CAD build for the part. Positions are in the model's coordinates, mm. A direction names the side the tool comes from. Coordinates: 2 decimals unless noted, no trailing zeros. Loops run counter-clockwise (first coordinate to the right, second up) from the corner with the lowest first, then second, coordinate; pieces in that order, holes last.
1) Saw through at A-A, the plane y = -285.75. Write the cut outline in (x, z).
2) Saw through at C-C, the plane z = -21.5. Write the cut outline in (x, y).
3) Two-plate mould, pull along X, no slides. Class faces 6 (the flat face through (-1, 304.8, 1)), 7 (the cylindrical face through (-66.86, -119.14, 12.52)), 8 (the flat face through (-95.25, -176, 16)): +X half, -X half, draft (parallel to the pull), parting line (faces both ways), or undercut.
4) Which spindle directions (+Z, -Z, +X, -X, +Y, -Y) get a long thin tool onto all of the face, cutting with end or side? Do faces 1 (the flat face through (-70, -92.075, 16)), 2 (the cylindrical face through (64.55, -122.16, 12.52)), 3 (the flat face through (95.25, -176, 16)), 4 (the flat face through (-118.269, 4, -25)), 5 (the flat face through (69, -257.175, 16)). Say none if no direction does.
5) Wall check: line 1 along Y through (x, z) = (57, 2); line 2 along X through (y, z) = (120, 1); line 3 along Y through (x, z) = (69.85, 19.75) (3 decimals). Give the ranges that are in metal, low to high.
6) Saw through at B-B, the plane x = -57.15. Write the cut outline in (y, z) (3 decimals), and give its area (3 significant figures).
7) Pin check, flat tips, straight feed: pin 1 Ø5 at (x, y) = (-37.5, -49.5) entering from +Z; pin 2 Ø21 at (x, z) = (59, 18) entering from -Y (3 decimals); pin 3 Ø15 at (y, z) = (-199.5, 15) entering from +X; pin 4 Ø14.5 at (x, y) = (69.85, -123.825) entering from +Z. Stop position of each tip, or through.
8) Saw through at D-D, the plane y = 93. Write the cut outline in (x, z), and give its area (3 significant figures).
```python
from build123d import *

# Parameters (mm, degrees)
F0_R     = 5.55625
F0_R_2   = 7.14375
F1_DEPTH = 6.35
F2_W     = 6.35
F2_H     = 609.6
F3_DEPTH = 50.8
F4_W     = 50.8
F4_H     = 165.1
F5_DEPTH = 19.05
F6_DEPTH = 25.4
F7_R     = 6.35
F8_DEPTH = 25.4


with BuildPart() as f1:
    # F0 (on Top) → F1 (new body)
    with BuildSketch(Plane.XY):
        Polygon((-124.61875, 304.8), (-124.61875, -304.8), (124.61875, -304.8), (124.61875, 304.8), (0, 304.8), align=None)
        with Locations((-69.85, -225.425)):
            Circle(F0_R, mode=Mode.SUBTRACT)
        with Locations((-69.85, -123.825)):
            Circle(F0_R, mode=Mode.SUBTRACT)
        with BuildLine():
            ThreePointArc((75.40625, -225.425), (69.85, -230.98125), (64.29375, -225.425))
            ThreePointArc((64.29375, -225.425), (69.85, -219.86875), (75.40625, -225.425))
        make_face(mode=Mode.SUBTRACT)
        with BuildLine():
            ThreePointArc((75.40625, -123.825), (69.85, -129.38125), (64.29375, -123.825))
            ThreePointArc((64.29375, -123.825), (69.85, -118.26875), (75.40625, -123.825))
        make_face(mode=Mode.SUBTRACT)
        with Locations((-57.15, 120.65)):
            Circle(F0_R_2, mode=Mode.SUBTRACT)
        with Locations((-57.15, 196.85)):
            Circle(F0_R_2, mode=Mode.SUBTRACT)
        with BuildLine():
            ThreePointArc((64.29375, 120.65), (57.15, 113.50625), (50.00625, 120.65))
            ThreePointArc((50.00625, 120.65), (57.15, 127.79375), (64.29375, 120.65))
        make_face(mode=Mode.SUBTRACT)
        with BuildLine():
            ThreePointArc((64.29375, 196.85), (57.15, 189.70625), (50.00625, 196.85))
            ThreePointArc((50.00625, 196.85), (57.15, 203.99375), (64.29375, 196.85))
        make_face(mode=Mode.SUBTRACT)
    extrude(amount=F1_DEPTH)

    # F2 (on face) → F3 (join)
    with BuildSketch(Plane(origin=(0, 0, 0), x_dir=(1, 0, 0), z_dir=(0, 0, -1))):
        with Locations((-121.44375, 0)):
            Rectangle(F2_W, F2_H)
        with Locations((121.44375, 0)):
            Rectangle(F2_W, F2_H)
    extrude(amount=F3_DEPTH)

    # F4 (on face) → F5 (join)
    with BuildSketch(Plane.XY.offset(6.35)):
        with Locations((-69.85, -174.625)):
            Rectangle(F4_W, F4_H)
        with Locations((69.85, -174.625)):
            Rectangle(F4_W, F4_H)
    extrude(amount=F5_DEPTH)

    # F6 (cut): faces of the model
    f6_faces = [f1.faces().sort_by_distance(p)[0] for p in [
        (-69.85, -123.825, 6.35),
        (-69.85, -225.425, 6.35),
        (69.85, -225.425, 6.35),
        (69.85, -123.825, 6.35),
    ]]
    extrude(f6_faces, amount=-F6_DEPTH, mode=Mode.SUBTRACT)

    # F7 (on face) → F8 (cut)
    with BuildSketch(Plane(origin=(0, 0, 0), x_dir=(1, 0, 0), z_dir=(0, 0, -1))):
        with Locations((-92.86875, 285.75)):
            Circle(F7_R)
        with Locations((92.86875, 285.75)):
            Circle(F7_R)
        with Locations((92.86875, -285.75)):
            Circle(F7_R)
        with Locations((-92.86875, -285.75)):
            Circle(F7_R)
    extrude(amount=-F8_DEPTH, mode=Mode.SUBTRACT)


solid = f1.part
```
Data:
1. outline: (-124.62, -50.8) - (-118.27, -50.8) - (-118.27, 0) - (-99.22, 0) - (-99.22, 6.35) - (-124.62, 6.35) - close; (-86.52, 0) - (86.52, 0) - (86.52, 6.35) - (-86.52, 6.35) - close; (99.22, 0) - (118.27, 0) - (118.27, -50.8) - (124.62, -50.8) - (124.62, 6.35) - (99.22, 6.35) - close
2. outline: (-124.62, -304.8) - (-118.27, -304.8) - (-118.27, 304.8) - (-124.62, 304.8) - close; (118.27, -304.8) - (124.62, -304.8) - (124.62, 304.8) - (118.27, 304.8) - close
3. face 6: draft
3. face 7: undercut
3. face 8: -X half
4. face 1: +Z, +X, -X, +Y
4. face 2: +Z, -Z
4. face 3: +Z, +X, +Y, -Y
4. face 4: -Z, +Y, -Y
4. face 5: +Z, +X, -X, -Y
5. line 1: y = -304.8 to 113.51, 127.79 to 189.71, 203.99 to 304.8
5. line 2: x = -124.62 to -64.26, -50.04 to 50.04, 64.26 to 124.62
5. line 3: y = -257.175 to -230.981, -219.869 to -129.381, -118.269 to -92.075
6. outline: (-304.8, 0) - (113.506, 0) - (113.506, 6.35) - (-92.075, 6.35) - (-92.075, 25.4) - (-257.175, 25.4) - (-257.175, 6.35) - (-304.8, 6.35) - close; (127.794, 0) - (189.706, 0) - (189.706, 6.35) - (127.794, 6.35) - close; (203.994, 0) - (304.8, 0) - (304.8, 6.35) - (203.994, 6.35) - close
6. area: 6,830 mm2
7. pin 1: stops at z = 6.35
7. pin 2: stops at y = -257.175
7. pin 3: stops at x = 95.25
7. pin 4: stops at z = 25.4
8. outline: (-124.62, -50.8) - (-118.27, -50.8) - (-118.27, 0) - (118.27, 0) - (118.27, -50.8) - (124.62, -50.8) - (124.62, 6.35) - (-124.62, 6.35) - close
8. area: 2,230 mm2
